Source: CAD feature listing. Evaluate the final solid. Frame: model axes, mm. Give positions to 0.01 mm unless a question says otherwise; leave off trailing zeros. Loops run counter-clockwise (first coordinate to the right, second up) from the corner with the lowest first, then second, coordinate; pieces in that order, holes last. Notation, with made-up numbers: M -12,-17 L 30,-17 A35 ccw 30,20 Z; hole C 24,45.25 d9. An arc over 180 degrees is marked long. Answer in a Markdown table with one row per item.
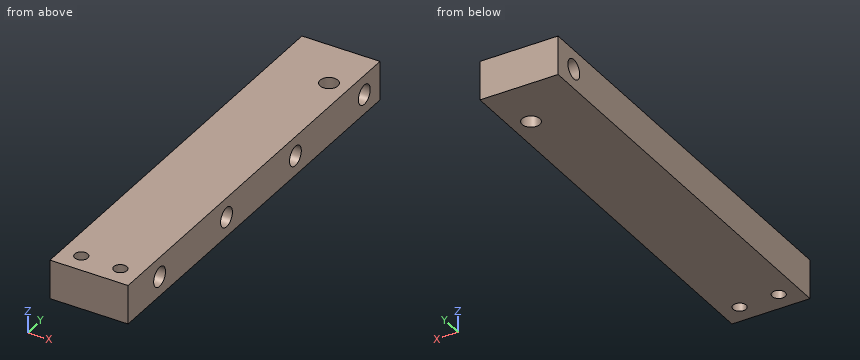
```python
from build123d import *

# Parameters (mm, degrees)
F0_W     = 38.1
F0_H     = 203.2
F1_DEPTH = 19.05
F2_R     = 4.7625
F3_DEPTH = 38.101
F4_R     = 3.175
F5_DEPTH = 19.051
F6_R     = 4.365625
F7_DEPTH = 19.051
F8_DEPTH = 12.7


with BuildPart() as f1:
    # F0 (on Top) → F1 (new body)
    with BuildSketch(Plane.XY):
        Rectangle(F0_W, F0_H)
    extrude(amount=F1_DEPTH)

    # F2 (on face) → F3 (cut, through all)
    with BuildSketch(Plane.YZ.offset(19.05)):
        with Locations((88.9, 9.525)):
            Circle(F2_R)
    extrude(amount=-F3_DEPTH, mode=Mode.SUBTRACT)

    # F4 (on face) → F5 (cut, through all)
    with BuildSketch(Plane.XY.offset(19.05)):
        with Locations((-9.525, -92.075)):
            Circle(F4_R)
        with Locations((9.525, -92.075)):
            Circle(F4_R)
    extrude(amount=-F5_DEPTH, mode=Mode.SUBTRACT)

    # F6 (on face) → F7 (cut, through all)
    with BuildSketch(Plane.XY.offset(19.05)):
        with Locations((9.525, 76.2)):
            Circle(F6_R)
    extrude(amount=-F7_DEPTH, mode=Mode.SUBTRACT)

    # F2 (on face) → F8 (cut)
    with BuildSketch(Plane.YZ.offset(19.05)):
        with Locations((33.3375, 9.525)):
            Circle(F2_R)
        with Locations((-22.225, 9.525)):
            Circle(F2_R)
        with Locations((-76.2, 9.525)):
            Circle(F2_R)
    extrude(amount=-F8_DEPTH, mode=Mode.SUBTRACT)


solid = f1.part
```
Q1. Section query B-B (x = 9). Give the number of separate pieces and of enclosed holes in the cut face, plus the area to 3 significant figures.
Values follow:
| item | result |
|---|---|
| separate pieces | 3 |
| enclosed holes | 4 |
| area | 3,300 mm^2 |
Q2. Section query C-C (z = 6.5). Output: boundary loops of the cut face in (x, y) (3 decimals), plus the area to 3 significant figures.
Values follow:
| item | result |
|---|---|
| outline | M -19.05,-101.6 L 19.05,-101.6 L 19.05,-79.878 L 6.35,-79.878 L 6.35,-72.522 L 19.05,-72.522 L 19.05,-25.903 L 6.35,-25.903 L 6.35,-18.547 L 19.05,-18.547 L 19.05,29.659 L 6.35,29.659 L 6.35,37.016 L 19.05,37.016 L 19.05,85.222 L -19.05,85.222 Z; M -19.05,92.578 L 19.05,92.578 L 19.05,101.6 L -19.05,101.6 Z; hole C -9.525,-92.075 d6.35; hole C 9.525,76.2 d8.731; hole C 9.525,-92.075 d6.35 |
| area | 7,060 mm^2 |
Q3. Section query A-A (y = 76.2). Output: boundary loops of the cut face in (x, z), plus the area to 3 significant figures.
Values follow:
| item | result |
|---|---|
| outline | M -19.05,0 L 5.16,0 L 5.16,19.05 L -19.05,19.05 Z; M 13.89,0 L 19.05,0 L 19.05,19.05 L 13.89,19.05 Z |
| area | 559 mm^2 |
Q4. Section query D-D (y = -76.2). Output: boundary loops of the cut face in (x, z).
Values follow:
| item | result |
|---|---|
| outline | M -19.05,0 L 19.05,0 L 19.05,4.76 L 6.35,4.76 L 6.35,14.29 L 19.05,14.29 L 19.05,19.05 L -19.05,19.05 Z |
Q5. Contact query for flat-ended pins moving along their axis: pin 1 Ø8.5 at (y, z) = (33.34, 9.52) entering from +X; pin 2 Ø6 at (x, y) = (0.5, 35) entering from -Z. Output: stop coordinate, or through.
Values follow:
| item | result |
|---|---|
| pin 1 | x = 6.35 |
| pin 2 | z = 0 |
Q6. Ray query, probe 1 along Y at (x, z) = (17.5, 9.75); probe 2 along X at (y, z) = (-92, 1); probe 3 along Y at (x, z) = (-7, 12.5). Return the intervals inside material, ascending. Write a range as from..to.
Values follow:
| item | result |
|---|---|
| probe 1 | -101.6..-80.96, -71.44..-26.98, -17.47..28.58, 38.09..84.14, 93.66..101.6 |
| probe 2 | -19.05..-12.7, -6.35..6.35, 12.7..19.05 |
| probe 3 | -101.6..-94, -90.15..85.18, 92.62..101.6 |
